Model file for the job. Use its own axes, mm. A direction names the side the tool comes from. Round coordinates to 2 decimals unless told otherwise and drop trailing zeros. Order: outer loops, then holes, each group sorted by start corner. A loop starts at its lowest first (then second) coordinate and runs counter-clockwise, first axis right, second up. Notation, with made-up numbers: M -37.75,-26 L 18.25,-26 A24 cw 18.25,5 Z; hole C 7,70 d5. An arc over 180 degrees is marked long. Return JSON: item names as keys, results as strings. Group by question number.
Item 1: Probe line 1 along Y through (x, z) = (0.5, -0.85); line 2 along X through (y, z) = (71, -1.05); line 3 along X through (y, z) = (48.5, 2.05). List the from-to ranges inside material, lowest first.
Item 2: Slice it at B-B on y = 58. Write the cut outline in (x, z).
Item 3: Which spindle directions (+Z, -Z, +X, -X, +Y, -Y) get a long thin tool onto all of the face, cutting with end or side? Do faces 1 (the face through (-18.71, 25.89, 0.04)), 2 (the face through (-3.1, -7, 0)). Say none if no direction does.
Item 4: Pin check, flat tips, straight feed: pin 1 Ø1.5 at (y, z) = (37, 1) entering from +X; pin 2 Ø1 at (x, z) = (-5, 2) entering from +Y. Stop position of each tip, or through.
Item 5: Pull direction Y, two halves, no side cores. Call faces 3 (the face through (-3.16, -7.63, -0.04)), 4 (the face through (38.34, 48.65, 0.04)), 5 (the face through (37.76, 48.5, -0.04)), 6 (the face through (-26.4, 47, -3)): pulls with the +Y half, pulls with the -Y half, needs draft (parallel to the pull), parting line crosses it, or undercut.
Item 6: Slice it at A-A on x = 0. Write the cut outline in (y, z).
Item 7: Slice it at C-C on z = 1.35. Write the cut outline in (x, y).
Autodesk Inventor part; units mm, degrees
ref_plane "Cross Section Plane" through (3.0943, -7.3315, 0) normal (0.9213, 0.3888, 0) x (0, 0, 1)
ref_plane "Work Plane2" through (0, 0, 0) normal (-1, 0, 0) x (0, 0, 1)
ref_plane "Work Plane3" through (0, 67, 0) normal (0.3476, -0.9376, 0) x (0, 0, 1)
sketch "Sketch Path" plane through (0, 0, 0) normal (0, 0, 1) x (1, 0, 0)
  arc A0 (-7.4354, -2.8355) -> (3.0943, -7.3315) centre (0, 0) ccw
  arc A1 (30.7005, 75.4079) -> (-29.7418, 55.6581) centre (0, 67) ccw
  arc A2 (39.275, 7.9388) -> (45.607, 20.9787) centre (34.9977, 18.0732) ccw
  line L0 (39.275, 7.9388) -> (3.0943, -7.3315)
  line L1 (-7.4354, -2.8355) -> (-29.7418, 55.6581)
  line L2 (30.7005, 75.4079) -> (45.607, 20.9787)
ref_plane "Cross Section Plane" through (3.0943, -7.3315, 0) normal (0.9213, 0.3888, 0) x (0, 0, 1)
ref_plane "Work Plane2" through (0, 0, 0) normal (-1, 0, 0) x (0, 0, 1)
ref_plane "Work Plane3" through (0, 67, 0) normal (0.3476, -0.9376, 0) x (0, 0, 1)
sketch "Cross Section" plane through (3.0943, -7.3315, 0) normal (0.9213, 0.3888, 0) x (0, 0, 1)
  line L0 (-3, 0.3) -> (3, 0.3)
  line L1 (3, 0.3) -> (3, -0.3)
  line L2 (3, -0.3) -> (-3, -0.3)
  line L3 (-3, -0.3) -> (-3, 0.3)
  line L4 (-3, 0) -> (3, 0) construction
  point P0 (0, 0)
  point P1 (0, 0)
  dimension "d0" = 6
  dimension "d4" = 0.3
  dimension "d5" = 0.3
sweep "Belt" add profiles "Cross Section" path "Sketch Path"
equation "\"d0\" = da_B"
equation "\"d4\" = da_a"
equation "\"d5\" = da_a2"
equation "\"da_B\" = 6"
equation "\"da_pb\" = 2.5"
equation "\"da_a\" = 0.3"
equation "\"da_S\" = 1.5"
equation "\"da_Beta\" = 20deg"
equation "\"da_Ht\" = 0.7"
equation "\"da_H\" = 1.3"
equation "\"da_a2\" = 0.3"
properties part number "Synchronous Belt" material "Rubber"
Output values:
{
 "1": {"line 1": "-8.24 to -7.64, 98.53 to 99.13", "line 2": "-31.88 to -31.28, 31.6 to 32.22", "line 3": "-27.33 to -26.69, 37.76 to 38.38"},
 "2": {"outline": "M -30.84,-3 L -30.22,-3 L -30.22,3 L -30.84,3 Z; M 35.16,-3 L 35.78,-3 L 35.78,3 L 35.16,3 Z"},
 "3": {"face 1": "+Z, -Z, -X, -Y", "face 2": "+Z, -Z"},
 "4": {"pin 1": "x = 41.74", "pin 2": "y = 98.81"},
 "5": {"face 3": "pulls with the -Y half", "face 4": "pulls with the +Y half", "face 5": "undercut", "face 6": "needs draft"},
 "6": {"outline": "M -8.26,-3 L -7.66,-3 L -7.66,3 L -8.26,3 Z; M 98.53,-3 L 99.13,-3 L 99.13,3 L 98.53,3 Z"},
 "7": {"outline": "M -30.02,55.55 L -7.72,-2.94 A8.26 ccw 3.21,-7.61 L 39.39,7.66 A11.3 ccw 45.9,21.06 L 30.99,75.49 A32.13 ccw long Z; hole M -29.46,55.76 L -7.16,-2.73 A7.66 ccw 2.98,-7.06 L 39.16,8.22 A10.7 ccw 45.32,20.9 L 30.41,75.33 A31.53 ccw long Z"}
}
